```python
from build123d import *

# Parameters (mm, degrees)
BOSS_EXTRUDE1_DEPTH     = 12.7
CUT_EXTRUDE1_DEPTH      = 73.765244725
CUT_EXTRUDE1_DEPTH_BACK = 73.765244725
SKETCH5_R               = 25.120382551


with BuildPart() as part:
    # Sketch4 → Boss-Extrude1 (new body)
    with BuildSketch(Plane(origin=(0, 0, 0), x_dir=(0, 0, -1), z_dir=(1, 0, 0))):
        Polygon((-47.071700205, -26.501749912), (-0.584661434, -54.016163133), (46.487038771, -27.514413221), (47.071700205, 26.501749912), (0.584661434, 54.016163133), (-46.487038771, 27.514413221), align=None)
    extrude(amount=BOSS_EXTRUDE1_DEPTH)

    # Sketch5 → Cut-Extrude1 (cut, two sides: drawn at the far end of the back side and taken through both)
    with BuildSketch(Plane(origin=(12.7, 0, 0), x_dir=(0, 0, -1), z_dir=(1, 0, 0)).offset(-CUT_EXTRUDE1_DEPTH_BACK)):
        Circle(SKETCH5_R)
    extrude(amount=CUT_EXTRUDE1_DEPTH + CUT_EXTRUDE1_DEPTH_BACK, mode=Mode.SUBTRACT)


solid = part.part
```
Input: part model. Units: mm. Frame: model coordinates. Give positions to 0.01 mm unless a question says otherwise; leave off trailing zeros. Order: outer loops, then holes, each group sorted by start corner. A loop starts at its lowest first (then second) coordinate and runs counter-clockwise, first axis right, second up. Notation, with made-up numbers: M 19,-25 L 42,-25 A26 cw 42,1 Z; hole C 37.5,-32 d1. An arc over 180 degrees is marked long. Return JSON: item names as keys, results as strings.
1) Section query B-B on z = 17. Output: boundary loops of the cut face in (x, y).
Taken from the geometry:
{"outline": "M 0,-44.3 L 12.7,-44.3 L 12.7,-18.49 L 0,-18.49 Z; M 0,18.49 L 12.7,18.49 L 12.7,44.12 L 0,44.12 Z"}
2) Section query D-D on z = -37.5. Output: boundary loops of the cut face in (x, y), and give its area (3 significant figures).
Taken from the geometry:
{"outline": "M 0,-32.57 L 12.7,-32.57 L 12.7,32.17 L 0,32.17 Z", "area": "822 mm2"}
3) Section query C-C on y = 0. Output: boundary loops of the cut face in (x, z).
Taken from the geometry:
{"outline": "M 0,-46.78 L 12.7,-46.78 L 12.7,-25.12 L 0,-25.12 Z; M 0,25.12 L 12.7,25.12 L 12.7,46.78 L 0,46.78 Z"}
4) Contact query for flat-ended pins moving along their axis: pin 1 (3 mm diameter, centred on x = 5, z = 25.5, fed in from +Y); pin 2 (3 mm diameter, centred on x = 7.5, z = -24.5, fed in from +Y); pin 3 (2 mm diameter, centred on x = 4.5, y = 25, fed in from -Z). Output: stop coordinate, or through.
Taken from the geometry:
{"pin 1": "stops at y = 40.17", "pin 2": "stops at y = 40.75", "pin 3": "stops at z = -47.07"}
5) Section query A-A on x = 1.75. Output: boundary loops of the cut face in (y, z).
Taken from the geometry:
{"outline": "M -54.02,0.58 L -27.51,-46.49 L 26.5,-47.07 L 54.02,-0.58 L 27.51,46.49 L -26.5,47.07 Z; hole C 0,0 d50.24"}
6) Line query: L1, parallel to Z at x = 7.75, y = 0; L2, parallel to Z at x = 5.25, y = 12; L3, parallel to Y at x = 6.25, z = 17. Output: solid intervals per line, ascending. Write a range as [from, to].
Taken from the geometry:
{"L1": "z = [-46.78, -25.12], [25.12, 46.78]", "L2": "z = [-46.91, -22.07], [22.07, 46.65]", "L3": "y = [-44.3, -18.49], [18.49, 44.12]"}
7) Mould query, pull axis Y, two halves, no side actions, for faces 1 (the face through (6.26, 40.95, 22.62)), 2 (the face through (0, -23.3, -9.8)), 3 (the face through (6.26, -40.07, 24.15)), 4 (the face through (6.26, -15.29, 19.93)). Classes: released by +Y, released by -Y, zero draft, split by the parting line, or undercut.
Taken from the geometry:
{"face 1": "released by +Y", "face 2": "zero draft", "face 3": "released by -Y", "face 4": "undercut"}
